Verification items for the finished model (mm, model axes). A direction names the side the tool comes from. Round coordinates to 2 decimals unless told otherwise and drop trailing zeros. Order: outer loops, then holes, each group sorted by start corner. A loop starts at its lowest first (then second) coordinate and runs counter-clockwise, first axis right, second up. Notation, with made-up numbers: (72, -19.5) -> (112, -19.5) arc R12 cw to (112, -0.5) -> close; hole circle Ø4 at (10.5, 28). An arc over 180 degrees is marked (long way). Return JSON: item names as keys, results as strings. Group by question number.
1) Section check C-C on x = 1. Enter the section's corners in (y, z), plus the area to 3 significant figures.
2) Tool access check on faces 4 (the flat face through (0, -22, -6.35)), 5 (the cylindrical face through (4.37, -9.66, -3.13)). Record the directions out of +Z, -Z, +X, -X, +Y, -Y that give a thin tool (end or side, any length) a straight path to the whole face; none if there is none.
3) Draft check along Y on faces 1 (the flat face through (0, -28, -3)), 2 (the flat face through (11, -4, -9)), 3 (the cylindrical face through (-1.08, -21.38, -3.13)). Enter one of: pulls with the +Y half, pulls with the -Y half, needs draft (parallel to the pull), parting line crosses it, or undercut.
4) Section check A-A on y = -16.5. Enter the section's corners in (x, z), plus the area to 3 significant figures.
5) Section check B-B on z = -12.5. Enter the section's corners in (x, y), plus the area to 3 significant figures.
6) Scan lines: L1, parallel to X at y = -4.25, z = -27.5; L2, parallel to Y at x = 0, z = -1.25; L3, parallel to Y at x = -9.25, z = -18.5. Record each from-to range of solid material in increasing order.
7) Depth check by flat-ended pin: pin 1 (2.5 mm diameter, centred on x = -7.5, z = -27.5, fed in from -Y); pin 2 (4.5 mm diameter, centred on x = 5.66, y = -10.84, fed in from -Z); pin 3 (4 mm diameter, centred on x = 1, z = -20, fed in from -Y). Enter the tip coordinate at first touch or a pass-through.
8) Section check D-D on x = 6.5. Enter the section's corners in (y, z), plus the area to 3 significant figures.
```python
from build123d import *

# Parameters (mm, degrees)
PAD_DEPTH         = 11
SKETCH002_R       = 5
SKETCH002_R_2     = 1.75
POCKET_DEPTH      = 34.001
POCKET_DEPTH_BACK = 0.001
SKETCH003_R       = 1.6
HOLE_DEPTH        = 28.001


with BuildPart() as part:
    # Sketch → Pad (new body, symmetric)
    with BuildSketch(Plane.YZ):
        Polygon((-28, 0), (0, 0), (0, -34), (-6.35, -34), (-6.35, -6.35), (-28, -6.35), align=None)
    extrude(amount=PAD_DEPTH, both=True)

    # Sketch002 → Pocket (cut, two sides)
    with BuildSketch(Plane.XY) as pocket_sk:
        with Locations((0, -16.5)):
            Circle(SKETCH002_R)
        with Locations((-5.656854, -22.156854)):
            Circle(SKETCH002_R_2)
        with Locations((5.656854, -22.156854)):
            Circle(SKETCH002_R_2)
        with Locations((5.656854, -10.843146)):
            Circle(SKETCH002_R_2)
        with Locations((-5.656854, -10.843146)):
            Circle(SKETCH002_R_2)
    extrude(amount=-POCKET_DEPTH, mode=Mode.SUBTRACT)
    extrude(pocket_sk.sketch, amount=POCKET_DEPTH_BACK, mode=Mode.SUBTRACT)

    # Sketch003 (on Face5 of Pocket) → Hole (cut, through all)
    with BuildSketch(Plane.ZX):
        with Locations((-27.5, 7.5)):
            Circle(SKETCH003_R)
        with Locations((-12.5, 7.5)):
            Circle(SKETCH003_R)
        with Locations((-12.5, -7.5)):
            Circle(SKETCH003_R)
        with Locations((-27.5, -7.5)):
            Circle(SKETCH003_R)
    extrude(amount=-HOLE_DEPTH, mode=Mode.SUBTRACT)


solid = part.part
```
Check result:
{
 "1": {"outline": "(-28, -6.35) -> (-21.4, -6.35) -> (-21.4, 0) -> (-28, 0) -> close; (-11.6, -6.35) -> (-6.35, -6.35) -> (-6.35, -34) -> (0, -34) -> (0, 0) -> (-11.6, 0) -> close", "area": "291 mm^2"},
 "2": {"face 4": "-Z, +X, -X, -Y", "face 5": "+Z, -Z"},
 "3": {"face 1": "pulls with the -Y half", "face 2": "needs draft", "face 3": "undercut"},
 "4": {"outline": "(-11, -6.35) -> (-5, -6.35) -> (-5, 0) -> (-11, 0) -> close; (5, -6.35) -> (11, -6.35) -> (11, 0) -> (5, 0) -> close", "area": "76.2 mm^2"},
 "5": {"outline": "(-11, -6.35) -> (-9.1, -6.35) -> (-9.1, 0) -> (-11, 0) -> close; (-5.9, -6.35) -> (5.9, -6.35) -> (5.9, 0) -> (-5.9, 0) -> close; (9.1, -6.35) -> (11, -6.35) -> (11, 0) -> (9.1, 0) -> close", "area": "99.1 mm^2"},
 "6": {"L1": "-11 to -9.1, -5.9 to 5.9, 9.1 to 11", "L2": "-28 to -21.5, -11.5 to 0", "L3": "-6.35 to 0"},
 "7": {"pin 1": "through", "pin 2": "z = -6.35", "pin 3": "y = -6.35"},
 "8": {"outline": "(-28, -6.35) -> (-23.69, -6.35) -> (-23.69, 0) -> (-28, 0) -> close; (-20.62, -6.35) -> (-12.38, -6.35) -> (-12.38, 0) -> (-20.62, 0) -> close; (-9.31, -6.35) -> (-6.35, -6.35) -> (-6.35, -11.25) -> (0, -11.25) -> (0, 0) -> (-9.31, 0) -> close; (-6.35, -34) -> (0, -34) -> (0, -28.75) -> (-6.35, -28.75) -> close; (-6.35, -26.25) -> (0, -26.25) -> (0, -13.75) -> (-6.35, -13.75) -> close", "area": "283 mm^2"}
}
